The listing builds one solid part. Answer for the finished solid, in the listing's coordinates (mm). A direction names the side the tool comes from. Round coordinates to 2 decimals unless told otherwise and drop trailing zeros. Write each loop counter-clockwise with the first axis right and the second up, starting at its lowest first coordinate (ties: lowest second). Pieces come first, ordered by that corner, then holes. Notation, with made-up numbers: M 32,84.5 L 53,84.5 A14 ccw 53,108.5 Z; hole C 12.25,-33 d6. An arc over 180 degrees is marked long. One line per item, written item: value. Start each with the question number.
(1) Consider probe 1 along X at (y, z) = (10.5, -8); probe 2 along Y at (x, z) = (-68, -15) (3 decimals); probe 3 along Z at (x, y) = (-28.5, 12). Determine where each line is inside the solid, lowest interval first.
(2) Given P1, Ø1, axis at x = -21.5, y = 45, coming from the +Z side; P2, Ø1.5, axis at x = -31.5, z = -26.5, coming from the +Y side (3 decimals); P3, Ø2, axis at y = 20.5, z = -17, coming from the +X side, each flat-ended and moving along its own axis, determine where each tip first touches the part or whether it passes through.
(3) For faces 1 (the flat face through (-40, 77.06, -63)), 2 (the flat face through (-35, 9.525, -29)), determine the directions among +Z, -Z, +X, -X, +Y, -Y from which every point of the face is accessible in a straight line to the end or side of a thin tool.
(4) Section B-B (z = -18) is taken. Determine the outline of the cut face in (x, y) (3 decimals), plus the area to 3 significant figures.
(5) Section A-A (x = -17.5) is taken. Determine the outline of the cut face in (y, z) (3 decimals), plus the area to 3 significant figures.
```python
from build123d import *

# Parameters (mm, degrees)
EXTRUDE1_DEPTH = 80.264
SKETCH2_W      = 57.737446173
SKETCH2_H      = 67.495663922
EXTRUDE2_DEPTH = 9.525


with BuildPart() as part:
    # Sketch1 → Extrude1 (new body)
    with BuildSketch(Plane(origin=(0, 0, 0), x_dir=(0, 0, -1), z_dir=(1, 0, 0))):
        Polygon((0, 0), (67.262446173, 0), (67.262446173, 77.060221675), (57.737446173, 77.060221675), (57.737446173, 9.525), (0, 9.525), align=None)
    extrude(amount=-EXTRUDE1_DEPTH)

    # Sketch2 → Extrude2 (add)
    with BuildSketch(Plane.ZY.offset(80.264)):
        with Locations((-28.868723087, 43.272831961)):
            Rectangle(SKETCH2_W, SKETCH2_H)
    extrude(amount=-EXTRUDE2_DEPTH)


solid = part.part
```
Recorded:
1. probe 1: x = -80.26 to -70.74
1. probe 2: y = 0 to 9.525
1. probe 3: z = -67.26 to -57.74
2. P1: stops at z = -57.74
2. P2: stops at y = 9.525
2. P3: stops at x = -70.74
3. face 1: +Z, -Z, +X, -X, +Y
3. face 2: +Z, +X, +Y
4. outline: M -80.264,0 L 0,0 L 0,9.525 L -70.739,9.525 L -70.739,77.021 L -80.264,77.021 Z
4. area: 1,410 mm2
5. outline: M 0,-67.262 L 77.06,-67.262 L 77.06,-57.737 L 9.525,-57.737 L 9.525,0 L 0,0 Z
5. area: 1,280 mm2
